Verification items for the finished model (mm, model axes). Face numbers are marked on the shaded views. A direction names the side the tool comes from. Round coordinates to 2 decimals unless told otherwise and drop trailing zeros. Write each loop counter-clockwise with the first axis right and the second up, starting at its lowest first coordinate (ties: lowest second). Pieces come first, ordered by that corner, then holes. Notation, with made-up numbers: M 56.5,-20.75 L 72.5,-20.75 A21 ccw 72.5,-16.75 Z; hole C -24,64 d1. An arc over 180 degrees is marked long. Answer in a Markdown table with one row per item. Add a question column.
1. Sectioned sample at B-B on z = 18. Record the cut outline in (x, y).
2. Sectioned sample at D-D on y = -32.5. Record the cut outline in (x, z).
3. Draft check along X on the marked faces 6, 7, 8 and 9. Enter one of: pulls with the +X half, pulls with the -X half, needs draft (parallel to the pull), parting line crosses it, or undercut.
4. Material ranges on probe 1 along X at (y, z) = (-9.5, 26); probe 2 along Y at (x, z) = (-27, 24); probe 3 along Z at (x, y) = (-26.6, -12.5), recorded low to high.
5. Set-up check for the marked faces 1, 2, 3, 4 and 5: record each of +Z, -Z, +X, -X, +Y, -Y from which the full face is reachable in a straight line by a thin tool's end or side.
6. Sectioned sample at A-A on y = -22.5. Record the cut outline in (x, z).
7. Sectioned sample at C-C on x = -35. Record the cut outline in (y, z).
8. Go/stop test with flat-tipped pins: pin 1 Ø9 at (y, z) = (-12.5, 24.81) entering from -X; pin 2 Ø4 at (x, y) = (-40, -17) entering from +Z; pin 3 Ø23 at (y, z) = (-17.5, 37.5) entering from +X; pin 4 Ø4 at (x, z) = (-21, 18) entering from +Y. Record where each tip stops, or that it passes through.
```python
from build123d import *

# Parameters (mm, degrees)
F1_DEPTH  = 35
F2_W      = 5.184
F2_H      = 10
F2_R      = 1.35
F3_DEPTH  = 5
F4_R      = 2.795
F5_DEPTH  = 5.5
F7_DEPTH  = 19
F8_R      = 1.35
F9_DEPTH  = 41.5
F10_DEPTH = 3.5


with BuildPart() as f1:
    # F0 (on Front) → F1 (new body)
    with BuildSketch(Plane.XZ):
        Polygon((-36.4558147092, 34.5085331884), (-36.4558147092, 19.1085331884), (-32.4558147092, 19.1085331884), (-32.4558147092, 30.5085331884), (-30.1558147092, 30.5085331884), (-30.1558147092, 12.0085331884), (-17.1558147092, 12.0085331884), (-17.1558147092, 17.0085331884), (-24.6558147092, 17.0085331884), (-24.6558147092, 34.5085331884), align=None)
    extrude(amount=F1_DEPTH)

    # F2 (on face) → F3 (join)
    with BuildSketch(Plane.XY.offset(17.0085331884)):
        with Locations((-19.7478147092, -5)):
            Rectangle(F2_W, F2_H)
        with Locations((-19.6558147092, -2.5)):
            Circle(F2_R, mode=Mode.SUBTRACT)
        with Locations((-19.7478147092, -30)):
            Rectangle(F2_W, F2_H)
        with Locations((-19.6558147092, -32.5)):
            Circle(F2_R, mode=Mode.SUBTRACT)
    extrude(amount=F3_DEPTH)

    # F4 (on face) → F5 (cut, through all)
    with BuildSketch(Plane.YZ.offset(-24.6558147092)):
        with Locations((-22.5, 24.8085331884)):
            Circle(F4_R)
        with Locations((-12.5, 24.8085331884)):
            Circle(F4_R)
    extrude(amount=-F5_DEPTH, mode=Mode.SUBTRACT)

    # F6 (on face) → F7 (join)
    with BuildSketch(Plane(origin=(0, 0, 0), x_dir=(-1, 0, 0), z_dir=(0, 1, 0))):
        Polygon((24.6558147092, 12.0085331884), (30.1558147092, 12.0085331884), (30.1558147092, 30.5085331884), (32.4558147092, 30.5085331884), (32.4558147092, 34.5085331884), (32.4558147092, 52.5085331884), (62.4558147092, 52.5085331884), (62.4558147092, 57.5085331884), (24.6558147092, 57.5085331884), align=None)
    extrude(amount=F7_DEPTH)

    # F8 (on face) → F9 (cut)
    with BuildSketch(Plane.XY.offset(57.5085331884)):
        with Locations((-26.9058147092, 4)):
            Circle(F8_R)
        with Locations((-26.9058147092, 15)):
            Circle(F8_R)
    extrude(amount=-F9_DEPTH, mode=Mode.SUBTRACT)

    # F10 (cut): faces of the model
    f10_faces = [f1.faces().sort_by_distance(p)[0] for p in [
        (-19.6558147092, -32.5, 17.0085331884),
        (-19.6558147092, -2.5, 17.0085331884),
    ]]
    extrude(f10_faces, amount=-F10_DEPTH, mode=Mode.SUBTRACT)


solid = f1.part
```
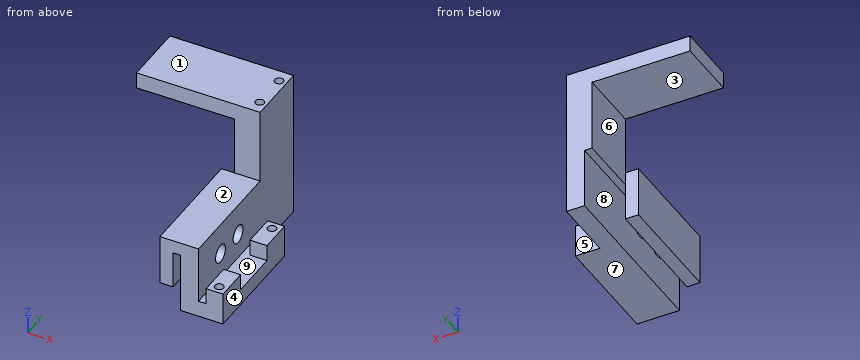
Geometry check:
| question | item | result |
|---|---|---|
| 1 | outline | M -30.16,-35 L -24.66,-35 L -24.66,19 L -30.16,19 Z; M -22.34,-35 L -17.16,-35 L -17.16,-25 L -22.34,-25 Z; M -22.34,-10 L -17.16,-10 L -17.16,0 L -22.34,0 Z; hole C -26.91,4 d2.7; hole C -26.91,15 d2.7; hole C -19.66,-32.5 d2.7; hole C -19.66,-2.5 d2.7 |
| 2 | outline | M -36.46,19.11 L -32.46,19.11 L -32.46,30.51 L -30.16,30.51 L -30.16,12.01 L -17.16,12.01 L -17.16,22.01 L -18.31,22.01 L -18.31,13.51 L -21.01,13.51 L -21.01,22.01 L -22.34,22.01 L -22.34,17.01 L -24.66,17.01 L -24.66,34.51 L -36.46,34.51 Z |
| 3 | face 6 | pulls with the -X half |
| 3 | face 7 | needs draft |
| 3 | face 8 | undercut |
| 3 | face 9 | undercut |
| 4 | probe 1 | x = -36.46 to -32.46, -30.16 to -24.66 |
| 4 | probe 2 | y = -35 to -25.18, -19.82 to -15.18, -9.82 to 2.65, 5.35 to 13.65, 16.35 to 19 |
| 4 | probe 3 | z = 12.01 to 22.01, 27.6 to 34.51 |
| 5 | face 1 | +Z, +X, -X, +Y, -Y |
| 5 | face 2 | +Z, +X, -X, -Y |
| 5 | face 3 | -Z, -X, +Y, -Y |
| 5 | face 4 | +Z, -Z, +X, +Y, -Y |
| 5 | face 5 | +Z, -Z, +X, +Y |
| 6 | outline | M -36.46,19.11 L -32.46,19.11 L -32.46,30.51 L -30.16,30.51 L -30.16,27.6 L -24.66,27.6 L -24.66,34.51 L -36.46,34.51 Z; M -30.16,12.01 L -17.16,12.01 L -17.16,17.01 L -24.66,17.01 L -24.66,22.01 L -30.16,22.01 Z |
| 7 | outline | M -35,19.11 L 0,19.11 L 0,34.51 L -35,34.51 Z; M 0,52.51 L 19,52.51 L 19,57.51 L 0,57.51 Z |
| 8 | pin 1 | stops at x = -36.46 |
| 8 | pin 2 | passes through |
| 8 | pin 3 | stops at x = -24.66 |
| 8 | pin 4 | stops at y = 0 |
